from build123d import *

# Parameters (mm, degrees)
BOSS_EXTRUDE1_DEPTH = 15
SKETCH5_R           = 4.4
CUT_EXTRUDE3_DEPTH  = 16
SKETCH3_W           = 16
SKETCH3_H           = 5
SKETCH3_W_2         = 2.5
SKETCH3_H_2         = 9
CUT_EXTRUDE4_DEPTH  = 52


with BuildPart() as part:
    # Sketch2 → Boss-Extrude1 (new body)
    with BuildSketch(Plane.XY):
        with BuildLine():
            Line((42.400497512, 28.014925373), (23.264667046, 28.014925373))
            ThreePointArc((23.264667046, 28.014925373), (21.639308303, 27.180347595), (21.370437848, 25.373134328))
            ThreePointArc((21.370437848, 25.373134328), (7.400497512, 5.889925373), (-6.569442823, 25.373134328))
            ThreePointArc((-6.569442823, 25.373134328), (-6.838313278, 27.180347595), (-8.463672021, 28.014925373))
            Line((-8.463672021, 28.014925373), (-27.599502488, 28.014925373))
            Line((-27.599502488, 28.014925373), (-27.599502488, -22.985074627))
            Line((-27.599502488, -22.985074627), (42.400497512, -22.985074627))
            Line((42.400497512, -22.985074627), (42.400497512, 28.014925373))
        make_face()
    extrude(amount=BOSS_EXTRUDE1_DEPTH)

    # Sketch5 → Cut-Extrude3 (cut, through all)
    with BuildSketch(Plane.XY.offset(15)):
        with Locations((7.400497512, -2.910074627)):
            Circle(SKETCH5_R)
    extrude(amount=-CUT_EXTRUDE3_DEPTH, mode=Mode.SUBTRACT)

    # Sketch3 → Cut-Extrude4 (cut, through all)
    with BuildSketch(Plane(origin=(0, 28.014925373, 0), x_dir=(1, 0, 0), z_dir=(0, 1, 0))):
        with Locations((-27.599502488, -7.5)):
            Rectangle(SKETCH3_W, SKETCH3_H)
        with Locations((42.400497512, -7.5)):
            Rectangle(SKETCH3_W, SKETCH3_H)
        with Locations((-19.599502488, -7.49995864)):
            Rectangle(SKETCH3_W_2, SKETCH3_H_2)
        with Locations((34.400497512, -7.5)):
            Rectangle(SKETCH3_W_2, SKETCH3_H_2)
    extrude(amount=-CUT_EXTRUDE4_DEPTH, mode=Mode.SUBTRACT)


solid = part.part
Input: part model. Units: mm. Frame: model coordinates. A direction names the side the tool comes from. Round coordinates to 2 decimals unless told otherwise and drop trailing zeros. Write each loop counter-clockwise with the first axis right and the second up, starting at its lowest first coordinate (ties: lowest second). Pieces come first, ordered by that corner, then holes.
1) Reachability of faces 4 (the flat face through (39, 3, 5)), 5 (the flat face through (-27.6, 3, 12)), 6 (the flat face through (34, 3, 12)) from +Z, -Z, +X, -X, +Y, -Y: full face, straight path, thin tool, end or side. Return the list, or none.
2) Contact query for a flat-ended pin moving along its axis: P1, Ø5.5, axis at x = 7.4, y = -2.91, coming from the +Z side. Output: stop coordinate, or through.
3) Cut plane D-D (y = 8). Return the cut outline in (x, z).
4) Cut plane A-A (z = 10.75). Return the cut outline in (x, y).
5) Cut plane C-C (y = -13.5). Return the cut outline in (x, z).
6) Draft query along X for faces 1 (the flat face through (42.4, 2, 12)), 2 (the flat face through (34, 3, 3)), 3 (the flat face through (7, 3, 0)). Return one class per face: pulls with the +X half, pulls with the -X half, needs draft (parallel to the pull), parting line crosses it, or undercut.
7) Cut plane B-B (x = 5.5). Return the cut outline in (y, z), then the cut area to 3 significant figures.
8) Ray query, L1, parallel to X at y = -15.5, z = 4.75; L2, parallel to Z at x = -22, y = 7; L3, parallel to Z at x = 35, y = -14. Return the intervals inside material, ascending.
Geometry says:
1. face 4: +X, +Y, -Y
1. face 5: +Z, -Z, -X, +Y, -Y
1. face 6: +Y, -Y
2. P1: passes through
3. outline: (-27.6, 0) - (-0.2, 0) - (-0.2, 15) - (-27.6, 15) - (-27.6, 10) - (-20.85, 10) - (-20.85, 12) - (-18.35, 12) - (-18.35, 3) - (-20.85, 3) - (-20.85, 5) - (-27.6, 5) - close; (15, 0) - (42.4, 0) - (42.4, 5) - (35.65, 5) - (35.65, 3) - (33.15, 3) - (33.15, 12) - (35.65, 12) - (35.65, 10) - (42.4, 10) - (42.4, 15) - (15, 15) - close
4. outline: (-27.6, -22.99) - (-20.85, -22.99) - (-20.85, 28.01) - (-27.6, 28.01) - close; (-18.35, -22.99) - (33.15, -22.99) - (33.15, 28.01) - (23.26, 28.01) arc R2 ccw to (21.37, 25.37) arc R14.75 cw (long way) to (-6.57, 25.37) arc R2 ccw to (-8.46, 28.01) - (-18.35, 28.01) - close; (35.65, -22.99) - (42.4, -22.99) - (42.4, 28.01) - (35.65, 28.01) - close; hole circle Ø8.8 at (7.4, -2.91)
5. outline: (-27.6, 0) - (42.4, 0) - (42.4, 5) - (35.65, 5) - (35.65, 3) - (33.15, 3) - (33.15, 12) - (35.65, 12) - (35.65, 10) - (42.4, 10) - (42.4, 15) - (-27.6, 15) - (-27.6, 10) - (-20.85, 10) - (-20.85, 12) - (-18.35, 12) - (-18.35, 3) - (-20.85, 3) - (-20.85, 5) - (-27.6, 5) - close
6. face 1: pulls with the +X half
6. face 2: undercut
6. face 3: needs draft
7. outline: (-22.99, 0) - (-6.88, 0) - (-6.88, 15) - (-22.99, 15) - close; (1.06, 0) - (6.01, 0) - (6.01, 15) - (1.06, 15) - close
7. area: 316 mm2
8. L1: x = -27.6 to -20.85, -18.35 to 33.15, 35.65 to 42.4
8. L2: z = 0 to 5, 10 to 15
8. L3: z = 0 to 3, 12 to 15
